For this review, use the dimensioned drawing (mm, ordinates from the lowest corner) and the shaded views. Give positions to 0.01 mm unless a question says otherwise; leave off trailing zeros. Loops run counter-clockwise (first coordinate to the right, second up) from the corner with the lowest first, then second, coordinate; pieces in that order, holes last. Notation, with made-up numbers: M -8,60.25 L 47,60.25 A26 cw 47,75.25 Z; hole C 9,32.5 d1. An arc over 180 degrees is marked long. Return JSON: item names as keys, results as strings.
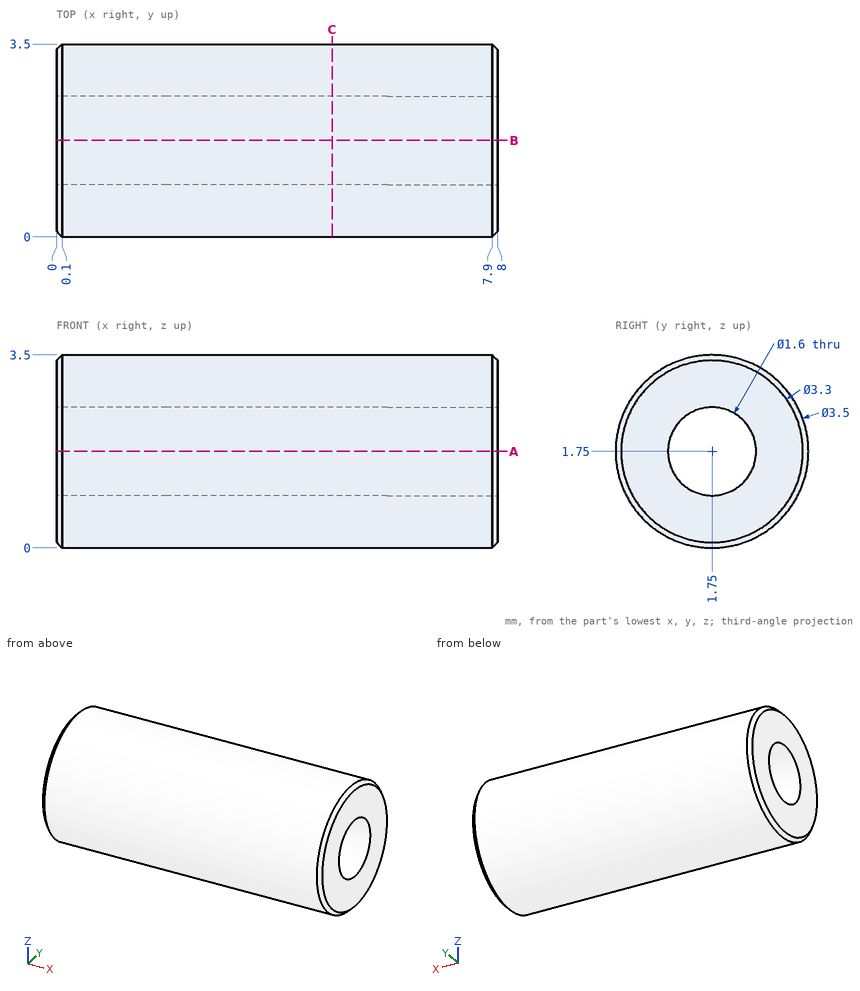
1) Consider section C-C on x = 5. Write out the cut boundary in (y, z).
From the geometry:
{"outline": "C 1.75,1.75 d3.5; hole C 1.75,1.75 d1.6"}
2) Consider section A-A on z = 1.75. Write out the cut boundary in (x, y), then the cut area to 3 significant figures.
From the geometry:
{"outline": "M 0,0.1 L 0.1,0 L 7.9,0 L 8,0.1 L 8,0.95 L 0,0.95 Z; M 0,2.55 L 8,2.55 L 8,3.4 L 7.9,3.5 L 0.1,3.5 L 0,3.4 Z", "area": "15.2 mm²"}
3) Insertion check: pin 1 (2 mm diameter, centred on x = 2, z = 1.5, fed in from +Y); pin 2 (1.5 mm diameter, centred on x = 2, y = 0.5, fed in from +Z); pin 3 (1.5 mm diameter, centred on x = 6.5, z = 0.5, fed in from +Y). Each pin has a flat end and moves straight along its axis. Give the tip position at first contact, or say it passes through.
From the geometry:
{"pin 1": "y = 3.5", "pin 2": "z = 3.43", "pin 3": "y = 3.43"}
4) Wall thickness on L1, parallel to Z at x = 1.2, y = 1.75; L2, parallel to Z at x = 5, y = 1.15; L3, parallel to Y at x = 1.75, z = 1.4: over which ranges is each line inside the solid? List them lowest first. Write a range as from..to.
From the geometry:
{"L1": "0..0.95, 2.55..3.5", "L2": "0.11..1.22, 2.28..3.39", "L3": "0.04..1.03, 2.47..3.46"}
